CAD build for the part. Positions are in the model's coordinates, mm. A direction names the side the tool comes from. Coordinates: 2 decimals unless noted, no trailing zeros. Order: outer loops, then holes, each group sorted by start corner. A loop starts at its lowest first (then second) coordinate and runs counter-clockwise, first axis right, second up. Notation, with made-up numbers: M 60.5,-6 L 119.5,-6 A5 cw 119.5,-2 Z; hole C 57,42 d2. An arc over 180 degrees is marked long. Write item = value, one per line.
from build123d import *

# Parameters (mm, degrees)
BOSS_EXTRUDE1_DEPTH = 18.3
FILLET1_R           = 2.54
SKETCH2_W           = 13.138787008
SKETCH2_H           = 9.53
SKETCH2_R           = 1.37
BOSS_EXTRUDE2_DEPTH = 2.1
FILLET2_R           = 1.27
SKETCH3_R           = 4
CUT_EXTRUDE1_DEPTH  = 14
SKETCH4_W           = 14.5
SKETCH4_H           = 7.1
SKETCH4_W_2         = 0.64
SKETCH4_H_2         = 0.64
CUT_EXTRUDE2_DEPTH  = 6.35


with BuildPart() as part:
    # Sketch1 → Boss-Extrude1 (new body)
    with BuildSketch(Plane.XY):
        with BuildLine():
            Line((15, 0), (15, -26.1))
            Line((15, -26.1), (-15, -26.1))
            Line((-15, -26.1), (-15, 0))
            ThreePointArc((-15, 0), (0, 15), (15, 0))
        make_face()
    extrude(amount=BOSS_EXTRUDE1_DEPTH)

    # Fillet1
    fillet1_edges = [part.edges().sort_by_distance(p)[0] for p in [
        (15, -13.05, 18.3),
        (0, 15, 18.3),
        (-15, -13.05, 18.3),
    ]]
    fillet(fillet1_edges, radius=FILLET1_R)

    # Sketch2 → Boss-Extrude2 (add)
    with BuildSketch(Plane(origin=(0, 0, 0), x_dir=(-1, 0, 0), z_dir=(0, 0, -1))):
        with Locations((19.030606496, 0)):
            Rectangle(SKETCH2_W, SKETCH2_H)
        with Locations((23, 0)):
            Circle(SKETCH2_R, mode=Mode.SUBTRACT)
        with Locations((-19.030606496, 0)):
            Rectangle(SKETCH2_W, SKETCH2_H)
        with Locations((-23, 0)):
            Circle(SKETCH2_R, mode=Mode.SUBTRACT)
    extrude(amount=-BOSS_EXTRUDE2_DEPTH)

    # Fillet2
    fillet2_edges = [part.edges().sort_by_distance(p)[0] for p in [
        (-25.6, -4.765, 1.05),
        (-25.6, 4.765, 1.05),
        (25.6, 4.765, 1.05),
        (25.6, -4.765, 1.05),
    ]]
    fillet(fillet2_edges, radius=FILLET2_R)

    # Sketch3 → Cut-Extrude1 (cut)
    with BuildSketch(Plane(origin=(0, 0, 0), x_dir=(-1, 0, 0), z_dir=(0, 0, -1))):
        Circle(SKETCH3_R)
    extrude(amount=-CUT_EXTRUDE1_DEPTH, mode=Mode.SUBTRACT)

    # Sketch4 → Cut-Extrude2 (cut)
    with BuildSketch(Plane.XZ.offset(26.1)):
        with Locations((0, 5.68)):
            Rectangle(SKETCH4_W, SKETCH4_H)
        with Locations((-5.08, 5.13)):
            Rectangle(SKETCH4_W_2, SKETCH4_H_2, mode=Mode.SUBTRACT)
        with Locations((-2.54, 5.13)):
            Rectangle(SKETCH4_W_2, SKETCH4_H_2, mode=Mode.SUBTRACT)
        with Locations((0, 5.13)):
            Rectangle(SKETCH4_W_2, SKETCH4_H_2, mode=Mode.SUBTRACT)
        with Locations((2.54, 5.13)):
            Rectangle(SKETCH4_W_2, SKETCH4_H_2, mode=Mode.SUBTRACT)
        with Locations((5.08, 5.13)):
            Rectangle(SKETCH4_W_2, SKETCH4_H_2, mode=Mode.SUBTRACT)
    extrude(amount=-CUT_EXTRUDE2_DEPTH, mode=Mode.SUBTRACT)


solid = part.part
(1) Wall check: line 1 (Y direction, x = -23, z = 0.75) (3 decimals); line 2 (Y direction, x = 0, z = 6.75); line 3 (Z direction, x = 6.5, y = -22). Give the ranges that are in metal, low to high. Write a range as from..to.
Evaluation:
line_1 = -4.765..-1.37, 1.37..4.765
line_2 = -19.75..-4, 4..15
line_3 = 0..2.13, 9.23..18.3
(2) Tool access for faces 1 (the face through (0, -23, 9.23)), 2 (the face through (-14.276, -12.867, 17.536)): list every direction of +Z, -Z, +X, -X, +Y, -Y with a clear straight run to the whole face (end or side of a thin tool).
Evaluation:
face_1 = -Y
face_2 = +Z, -X, +Y, -Y
(3) Slice it at A-A, the plane x = -23. Write the cut outline in (y, z) (3 decimals), then the cut area to 3 significant figures.
Evaluation:
outline = M -4.765,0 L -1.37,0 L -1.37,2.1 L -4.765,2.1 Z; M 1.37,0 L 4.765,0 L 4.765,2.1 L 1.37,2.1 Z
area = 14.3 mm²
(4) Slice it at C-C, the plane y = -15. Write the cut outline in (x, z).
Evaluation:
outline = M -15,0 L 15,0 L 15,15.76 A2.54 ccw 12.46,18.3 L -12.46,18.3 A2.54 ccw -15,15.76 Z
(5) Pin check, flat tips, straight feed: pin 1 Ø10 at (y, z) = (-3, 13.5) entering from -X; pin 2 Ø0.6 at (x, z) = (17, 1) entering from +Y (3 decimals); pin 3 Ø3.5 at (x, y) = (-23, 0) entering from +Z. Stop position of each tip, or through.
Evaluation:
pin_1 = -15
pin_2 = 4.765
pin_3 = 2.1
(6) Slice it at D-D, the plane x = 17. Write the cut outline in (y, z) (3 decimals).
Evaluation:
outline = M -4.765,0 L 4.765,0 L 4.765,2.1 L -4.765,2.1 Z
(7) Pull direction Y, two halves, no side cores. Call faces 3 (the face through (19, 4.765, 1)), 4 (the face through (20, 0, 2.1)), 5 (the face through (0.867, -3.905, 6.902)): +Y half, -Y half, draft (parallel to the pull), parting line (faces both ways), or undercut.
Evaluation:
face_3 = +Y half
face_4 = draft
face_5 = undercut
(8) Slice it at B-B, the plane z = 8.5. Write the cut outline in (x, y).
Evaluation:
outline = M -15,-26.1 L -7.25,-26.1 L -7.25,-19.75 L 7.25,-19.75 L 7.25,-26.1 L 15,-26.1 L 15,0 A15 ccw -15,0 Z; hole C 0,0 d8
